from build123d import *

# Parameters (mm, degrees)
SKETCH1_R           = 2.0828
BOSS_EXTRUDE1_DEPTH = 3.175
FILLET1_R           = 3.175


with BuildPart() as part:
    # Sketch1 → Boss-Extrude1 (new body)
    with BuildSketch(Plane(origin=(0, 0, 0), x_dir=(1, 0, 0), z_dir=(0, 1, 0))):
        with BuildLine():
            Line((-15.950085837, 2.921), (-18.3111574, 2.921))
            Line((-18.3111574, 2.921), (-18.3111574, 9.371))
            Line((-18.3111574, 9.371), (-15.1361574, 9.371))
            Line((-15.1361574, 9.371), (-15.1361574, 12.546))
            Line((-15.1361574, 12.546), (-13.204371576, 12.546))
            Line((-13.204371576, 12.546), (-3.831834579, 12.546))
            ThreePointArc((-3.831834579, 12.546), (2.162458915, 17.20722233), (8.338892533, 12.790185329))
            Line((8.338892533, 12.790185329), (12.221790763, 4.5085))
            Line((12.221790763, 4.5085), (12.221790763, 2.921))
            Line((12.221790763, 2.921), (6.35, 2.921))
            Line((6.35, 2.921), (6.35, -2.921))
            Line((6.35, -2.921), (-6.35, -2.921))
            Line((-6.35, -2.921), (-6.35, 2.921))
            Line((-6.35, 2.921), (-15.950085837, 2.921))
        make_face()
        with Locations(Location((2.289835434, 10.8585, 0), (0, 0, 270))):
            Circle(SKETCH1_R, mode=Mode.SUBTRACT)
    extrude(amount=BOSS_EXTRUDE1_DEPTH)

    # Fillet1
    fillet1_edges = [part.edges().sort_by_distance(p)[0] for p in [
        (-3.831834579, 1.5875, -12.546),
        (12.221790763, 1.5875, -4.5085),
    ]]
    fillet(fillet1_edges, radius=FILLET1_R)


solid = part.part
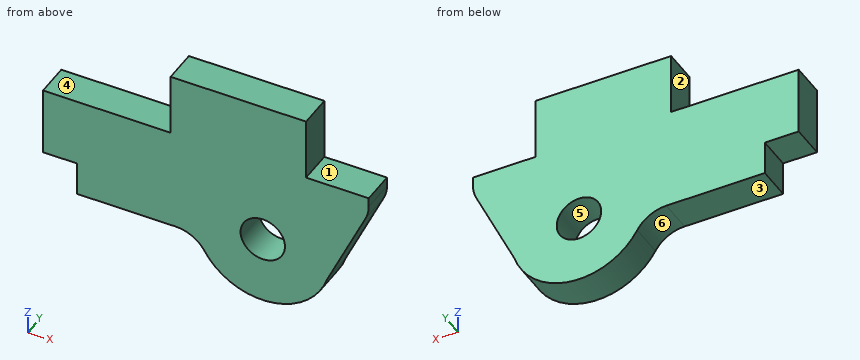
Design review of the part built by this model. Coordinates are the model's own, in mm. Face numbers are marked on the shaded views. A direction names the side the tool comes from. Give positions to 0.01 mm unless a question says otherwise; leave off trailing zeros. Loops run counter-clockwise (first coordinate to the right, second up) from the corner with the lowest first, then second, coordinate; pieces in that order, holes last. Notation, with made-up numbers: (82, 58) - (90, 58) arc R24 ccw to (90, 79) - close; hole circle Ø3 at (39, -25.5). An arc over 180 degrees is marked (long way). Use CSV: the item, a comma, the result in double quotes. Start each with the question number.
1. Insertion check: P1, Ø1.6, axis at x = -12, y = 1.5, coming from the +Z side; P2, Ø1.6, axis at y = 1.5, z = 0.5, coming from the -X side. Each pin has a flat end and moves straight along its axis. Give the tip position at first contact, or say it passes through.
2. Add section A-A (z = -10). State the section outline as (x, y) points (3 decimals).
3. Draft analysis for pull direction X (two halves, no side actions). For the marked faces 4, 5 and 6, state which applies: released by +X, released by -X, zero draft, split by the parting line, or undercut.
4. Add section D-D (x = -12). State the section outline as (y, z) points (3 decimals).
5. Wall thickness on L1, parallel to X at y = 2.8, z = -0.75; L2, parallel to X at y = 0.25, z = -10.75; L3, parallel to Z at x = -15, y = 2.95: over which ranges is each line inside the solid? List them lowest first.
6. Machinability: for the marked faces 1, 2 and 3, which of the approach directions +Z, -Z, +X, -X, +Y, -Y give a long, thin tool a straight path to every point of the face, cutting with its end or side? Answer none if there is none.
7. Add section C-C (x = 4). State the section outline as (y, z) points (3 decimals).
Results found:
1,P1,"stops at z = -2.92"
1,P2,"stops at x = -6.35"
2,outline,"(-15.136, 0) - (0.392, 0) - (0.392, 3.175) - (-15.136, 3.175) - close; (4.187, 0) - (9.647, 0) - (9.647, 3.175) - (4.187, 3.175) - close"
3,face 4,"zero draft"
3,face 5,"undercut"
3,face 6,"released by -X"
4,outline,"(0, -12.546) - (3.175, -12.546) - (3.175, -2.921) - (0, -2.921) - close"
5,L1,"x = -6.35 to 6.35"
5,L2,"x = -15.14 to 0.21, 4.37 to 9.3"
5,L3,"z = -12.55 to -2.92"
6,face 1,"+Z, +X, +Y, -Y"
6,face 2,"+Z, -X, +Y, -Y"
6,face 3,"-Z, -X, +Y, -Y"
7,outline,"(0, -16.974) - (3.175, -16.974) - (3.175, -12.047) - (0, -12.047) - close; (0, -9.67) - (3.175, -9.67) - (3.175, 2.921) - (0, 2.921) - close"
